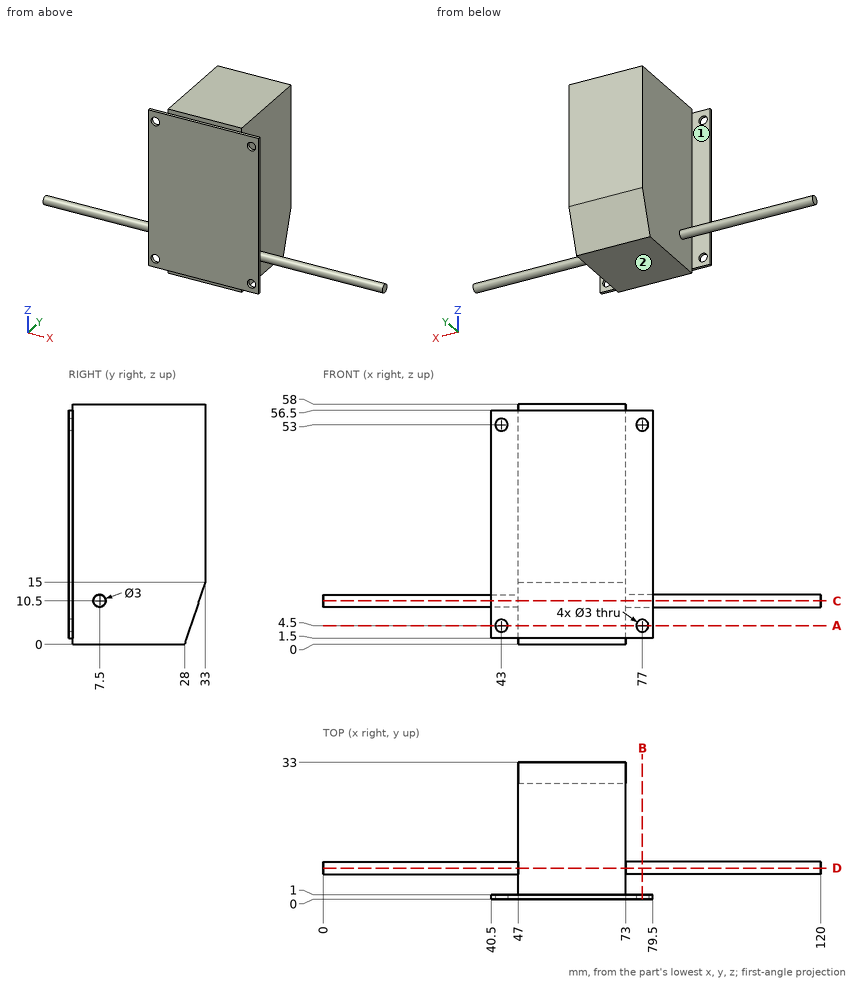
Geometry check sheet. Reference: drawing and pictorial views, mm from the part's lowest x, y, z. A direction names the side the tool comes from. Round coordinates to 2 decimals unless told otherwise and drop trailing zeros. Order: outer loops, then holes, each group sorted by start corner. A loop starts at its lowest first (then second) coordinate and runs counter-clockwise, first axis right, second up. Notation, with made-up numbers: M 28,8.5 L 80,8.5 A26 cw 80,32.5 Z; hole C 88,64.25 d5. An arc over 180 degrees is marked long. Answer in a Markdown table with one row per item.
(1) Scan lines: probe 1 along Z at (x, y) = (77, 0.35); probe 2 along X at (y, z) = (0.45, 4.5); probe 3 along X at (y, z) = (25.5, 29.5). Record each from-to range of solid material in increasing order. Write a range as from..to.
Responses:
| item | result |
|---|---|
| probe 1 | z = 1.5..3, 6..51.5, 54.5..56.5 |
| probe 2 | x = 40.5..41.5, 44.5..75.5, 78.5..79.5 |
| probe 3 | x = 47..73 |
(2) Sectioned sample at B-B, the plane x = 77. Record the cut outline in (y, z), and give its area (3 significant figures).
Responses:
| item | result |
|---|---|
| outline | M 0,1.5 L 1,1.5 L 1,3 L 0,3 Z; M 0,6 L 1,6 L 1,51.5 L 0,51.5 Z; M 0,54.5 L 1,54.5 L 1,56.5 L 0,56.5 Z; C 7.5,10.5 d3 |
| area | 56.1 mm² |
(3) Tool access check on the marked faces 1 and 2. Record the directions out of +Z, -Z, +X, -X, +Y, -Y that give a thin tool (end or side, any length) a straight path to the whole face; none if there is none.
Responses:
| item | result |
|---|---|
| face 1 | +Z, -Z, -X |
| face 2 | -Z, +X, -X, +Y, -Y |
(4) Sectioned sample at A-A, the plane z = 4.5. Record the cut outline in (x, y).
Responses:
| item | result |
|---|---|
| outline | M 40.5,0 L 41.5,0 L 41.5,1 L 40.5,1 Z; M 44.5,0 L 75.5,0 L 75.5,1 L 73,1 L 73,29.5 L 47,29.5 L 47,1 L 44.5,1 Z; M 78.5,0 L 79.5,0 L 79.5,1 L 78.5,1 Z |
(5) Go/stop test with flat-tipped pins: P1, Ø3.5, axis at x = 77, z = 53, coming from the +Y side; P2, Ø1, axis at y = 12, z = 10, coming from the +X side; P3, Ø6, axis at x = 84, y = 4, coming from the +Z side. Record where each tip stops, or that it passes through.
Responses:
| item | result |
|---|---|
| P1 | stops at y = 1 |
| P2 | stops at x = 73 |
| P3 | stops at z = 11.91 |
(6) Sectioned sample at C-C, the plane z = 10.5. Record the cut outline in (x, y), and give its area (3 significant figures).
Responses:
| item | result |
|---|---|
| outline | M 0,6 L 47,6 L 47,1 L 40.5,1 L 40.5,0 L 79.5,0 L 79.5,1 L 73,1 L 73,6 L 120,6 L 120,9 L 73,9 L 73,31.5 L 47,31.5 L 47,9 L 0,9 Z |
| area | 1,110 mm² |
(7) Sectioned sample at D-D, the plane y = 7.5. Record the cut outline in (x, z).
Responses:
| item | result |
|---|---|
| outline | M 0,9 L 47,9 L 47,0 L 73,0 L 73,9 L 120,9 L 120,12 L 73,12 L 73,58 L 47,58 L 47,12 L 0,12 Z |
